Geometry: see drawing. Coordinates: mm, zero at the bounding-box minimum. A direction names the side the tool comes from. Give positions to 0.01 mm unless a question says otherwise; leave off trailing zeros. Write each loop counter-clockwise with the first axis right and the second up, starting at its lowest first coordinate (ties: lowest second). Pieces come first, ordered by that corner, then holes. Notation, with made-up numbers: (30.5, 46.25) - (75.5, 46.25) arc R17 ccw to (75.5, 79.25) - close; hole circle Ø7 at (37, 3.5). An arc over 180 degrees is marked (long way). Use a Markdown table: item, result. Add a question column.
1. Section query B-B, the plane x = 44.5. Return loops of the section in (y, z), plus the area to 3 significant figures.
2. Mould query, pull axis Y, two halves, no side actions, for the marked faces 3, 4 and 5. Classes: released by +Y, released by -Y, zero draft, split by the parting line, or undercut.
3. Pin query (flat end, axial travel): pin 1 (10 mm diameter, centred on x = 38, z = 14.5, fed in from -Y); pin 2 (7.5 mm diameter, centred on x = 14, y = 22.5, fed in from -Z); pin 3 (5.5 mm diameter, centred on x = 32.5, z = 8, fed in from +Y). Return the tip coordinate at first contact, or that it passes through.
4. Set-up query: the marked faces 1 and 2. Return all of +Z, -Z, +X, -X, +Y, -Y with unobstructed straight access to the full face (end or side cutting, diameter ignored); none if empty.
5. Section query D-D, the plane y = 13.5. Count the separate pieces of the cut face and the enclosed holes in it, plus the area to 3 significant figures.
6. Section query C-C, the plane z = 14.25. Return loops of the section in (x, y), plus the area to 3 significant figures.
7. Section query A-A, the plane y = 17.78. Return loops of the section in (x, z).
8. Material intervals for probe 1 along X at (y, z) = (17.78, 15); probe 2 along X at (y, z) = (22.5, 17); probe 3 along Y at (x, z) = (6, 9.5), sorted ascending.
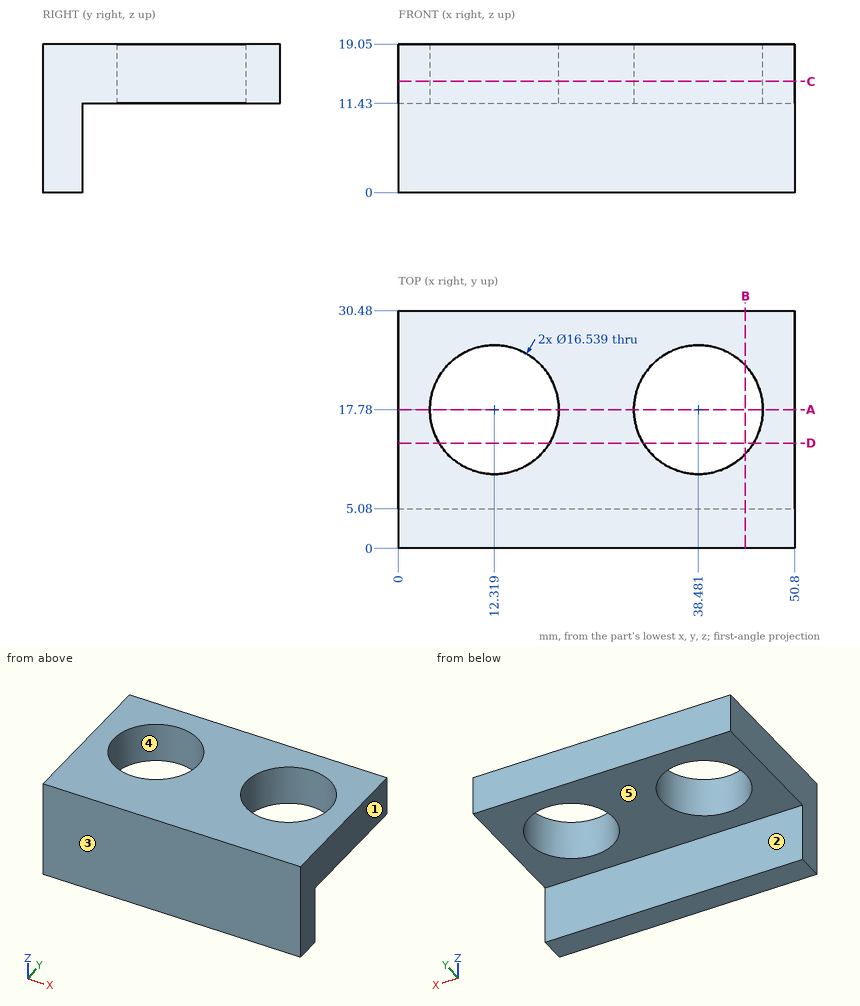
Result sheet:
| question | item | result |
|---|---|---|
| 1 | outline | (0, 0) - (5.08, 0) - (5.08, 11.43) - (12.11, 11.43) - (12.11, 19.05) - (0, 19.05) - close; (23.45, 11.43) - (30.48, 11.43) - (30.48, 19.05) - (23.45, 19.05) - close |
| 1 | area | 204 mm² |
| 2 | face 3 | released by -Y |
| 2 | face 4 | undercut |
| 2 | face 5 | zero draft |
| 3 | pin 1 | stops at y = 0 |
| 3 | pin 2 | stops at z = 11.43 |
| 3 | pin 3 | stops at y = 5.08 |
| 4 | face 1 | +Z, -Z, +X, +Y, -Y |
| 4 | face 2 | -Z, +X, -X, +Y |
| 5 | separate pieces | 3 |
| 5 | enclosed holes | 0 |
| 5 | area | 171 mm² |
| 6 | outline | (0, 0) - (50.8, 0) - (50.8, 30.48) - (0, 30.48) - close; hole circle Ø16.54 at (12.32, 17.78); hole circle Ø16.54 at (38.48, 17.78) |
| 6 | area | 1,120 mm² |
| 7 | outline | (0, 11.43) - (4.05, 11.43) - (4.05, 19.05) - (0, 19.05) - close; (20.59, 11.43) - (30.21, 11.43) - (30.21, 19.05) - (20.59, 19.05) - close; (46.75, 11.43) - (50.8, 11.43) - (50.8, 19.05) - (46.75, 19.05) - close |
| 8 | probe 1 | x = 0 to 4.05, 20.59 to 30.21, 46.75 to 50.8 |
| 8 | probe 2 | x = 0 to 5.53, 19.11 to 31.69, 45.27 to 50.8 |
| 8 | probe 3 | y = 0 to 5.08 |
